```python
from build123d import *

# Parameters (mm, degrees)
SKETCH_W      = 13
SKETCH_H      = 10
PAD_DEPTH     = 1.6
SKETCH001_R   = 1.5
SKETCH001_W   = 0.65
SKETCH001_H   = 0.65
POCKET_DEPTH  = 5
SKETCH002_W   = 2.6
SKETCH002_H   = 2.6
PAD001_DEPTH  = 0.03
SKETCH003_W   = 2.1
SKETCH003_H   = 2.1
PAD002_DEPTH  = 0.9
FILLET_R      = 0.3
FILLET001_R   = 0.05
FILLET002_R   = 0.2
SKETCH004_W   = 1.1
SKETCH004_H   = 2
SKETCH004_W_2 = 1.5
SKETCH004_H_2 = 0.9
SKETCH004_H_3 = 0.75
SKETCH004_H_4 = 2.9
SKETCH004_W_3 = 3.2
SKETCH004_H_5 = 1.4
SKETCH004_W_4 = 0.8
SKETCH004_H_6 = 1.6
PAD003_DEPTH  = 0.27


with BuildPart() as part:
    # Sketch → Pad (new body)
    with BuildSketch(Plane.XY):
        with Locations((6.5, 5)):
            Rectangle(SKETCH_W, SKETCH_H)
    extrude(amount=PAD_DEPTH)

    # Sketch001 → Pocket (cut)
    with BuildSketch(Plane.XY):
        with Locations((10.4, 7.6)):
            Circle(SKETCH001_R)
        with Locations((1.4, 8.6)):
            Rectangle(SKETCH001_W, SKETCH001_H)
        with Locations((1.4, 6.2)):
            Rectangle(SKETCH001_W, SKETCH001_H)
        with Locations((1.4, 3.8)):
            Rectangle(SKETCH001_W, SKETCH001_H)
        with Locations((1.4, 1.4)):
            Rectangle(SKETCH001_W, SKETCH001_H)
    extrude(amount=POCKET_DEPTH, mode=Mode.SUBTRACT)

    # Sketch002 (on Face5 of Pocket) → Pad001 (join)
    with BuildSketch(Plane.XY.offset(1.6)):
        with Locations((10.6, 2.7)):
            Rectangle(SKETCH002_W, SKETCH002_H)
    extrude(amount=PAD001_DEPTH)

    # Sketch003 (on Face28 of Pad001) → Pad002 (join)
    with BuildSketch(Plane.XY.offset(1.63)):
        with Locations((10.6, 2.7)):
            Rectangle(SKETCH003_W, SKETCH003_H)
    extrude(amount=PAD002_DEPTH)

    # Fillet
    fillet_edges = [part.edges().sort_by_distance(p)[0] for p in [
        (9.55, 1.65, 2.08),
        (9.55, 3.75, 2.08),
        (11.65, 1.65, 2.08),
        (11.65, 3.75, 2.08),
    ]]
    fillet(fillet_edges, radius=FILLET_R)

    # Fillet001
    fillet001_edges = [part.edges().sort_by_distance(p)[0] for p in [
        (9.637868, 1.737868, 1.63),
    ]]
    fillet(fillet001_edges, radius=FILLET001_R)

    # Fillet002
    fillet002_edges = [part.edges().sort_by_distance(p)[0] for p in [
        (10.6, 1.65, 2.53),
    ]]
    fillet(fillet002_edges, radius=FILLET002_R)

    # Sketch004 (on Face53 of Fillet002) → Pad003 (join)
    with BuildSketch(Plane(origin=(0, 0, 0), x_dir=(1, 0, 0), z_dir=(0, 0, -1))):
        with Locations((5.65, -2.1)):
            Rectangle(SKETCH004_W, SKETCH004_H)
        with Locations((8.7, -1.35)):
            Rectangle(SKETCH004_W_2, SKETCH004_H_2)
        with Locations((8.7, -2.95)):
            Rectangle(SKETCH004_W_2, SKETCH004_H_2)
        with Locations((8.7, -4.425)):
            Rectangle(SKETCH004_W_2, SKETCH004_H_3)
        with Locations((5.85, -7.65)):
            Rectangle(SKETCH004_W, SKETCH004_H_4)
        with Locations((4.8, -4.8)):
            Rectangle(SKETCH004_W_3, SKETCH004_H_5)
        with Locations((3.3, -8)):
            Rectangle(SKETCH004_W_4, SKETCH004_H_6)
    extrude(amount=PAD003_DEPTH)


with BuildPart() as part_1:
    # Body placement: moved
    add(part.part.moved(Location((0, 0, 1))))


solid = part_1.part
```
Geometry: final body of the model. Coordinates: model frame, mm. Round coordinates to 2 decimals unless told otherwise and drop trailing zeros. Order: outer loops, then holes, each group sorted by start corner. A loop starts at its lowest first (then second) coordinate and runs counter-clockwise, first axis right, second up. Notation, with made-up numbers: M 75.5,29.25 L 133.5,29.25 A31 ccw 133.5,65.25 Z; hole C 59.25,87.25 d3. An arc over 180 degrees is marked long. Use one line per item in the form item = value. Start each with the question number.
Q1. Cut plane B-B (z = 2.05). Return loops of the section in (x, y) (3 decimals).
Q2. Mould query, pull axis Y, two halves, no side actions, for faces 1 (the face through (9.29, 8.61, 1.79)), 2 (the face through (6, 8, 0.73)), 3 (the face through (6, 10, 2)). Classes: +Y half, -Y half, draft (parallel to the pull), parting line (faces both ways), or undercut.
Q3. Pin query (flat end, axial travel): pin 1 Ø3 at (x, y) = (3, 8) entering from +Z. Return the tip coordinate at first contact, or that it passes through.
Q4. Cut plane D-D (x = 7). Return loops of the section in (y, z), and give its area (3 significant figures).
Q5. Cut plane A-A (y = 7.6). Return loops of the section in (x, z).
Q6. Material intervals for line 1 (Y direction, x = 10.4, z = 2); line 2 (X direction, y = 7.6, z = 1.8); line 3 (Z direction, x = 3.25, y = 7.25), sorted ascending. Write a range as [from, to].
Geometry results:
q1.outline = M 0,0 L 13,0 L 13,10 L 0,10 Z; hole M 1.075,1.075 L 1.725,1.075 L 1.725,1.725 L 1.075,1.725 Z; hole M 1.075,3.475 L 1.725,3.475 L 1.725,4.125 L 1.075,4.125 Z; hole M 1.075,5.875 L 1.725,5.875 L 1.725,6.525 L 1.075,6.525 Z; hole M 1.075,8.275 L 1.725,8.275 L 1.725,8.925 L 1.075,8.925 Z; hole C 10.4,7.6 d3
q2.face_1 = undercut
q2.face_2 = draft
q2.face_3 = +Y half
q3.pin_1 = 2.6
q4.outline = M 0,1 L 10,1 L 10,2.6 L 0,2.6 Z
q4.area = 16.0 mm^2
q5.outline = M 0,1 L 2.9,1 L 2.9,0.73 L 3.7,0.73 L 3.7,1 L 5.3,1 L 5.3,0.73 L 6.4,0.73 L 6.4,1 L 8.9,1 L 8.9,2.6 L 0,2.6 Z; M 11.9,1 L 13,1 L 13,2.6 L 11.9,2.6 Z
q6.line_1 = [0, 6.1], [9.1, 10]
q6.line_2 = [0, 8.9], [11.9, 13]
q6.line_3 = [0.73, 2.6]
